from build123d import *

# Parameters (mm, degrees)
SKETCH1_W               = 72
SKETCH1_H               = 64
BOSS_EXTRUDE1_DEPTH     = 2.5
SKETCH2_R               = 3
BOSS_EXTRUDE2_DEPTH     = 11
CUT_EXTRUDE1_DEPTH      = 51.02249494
CUT_EXTRUDE1_DEPTH_BACK = 51.02249494
SKETCH3_R               = 1.5
FILLET1_R               = 5


with BuildPart() as part:
    # Sketch1 → Boss-Extrude1 (new body)
    with BuildSketch(Plane(origin=(0, 0, 0), x_dir=(1, 0, 0), z_dir=(0, 1, 0))):
        Rectangle(SKETCH1_W, SKETCH1_H)
    extrude(amount=BOSS_EXTRUDE1_DEPTH)

    # Sketch2 → Boss-Extrude2 (add)
    with BuildSketch(Plane(origin=(0, 2.5, 0), x_dir=(1, 0, 0), z_dir=(0, 1, 0))):
        with Locations(Location((-31, 27, 0), (0, 0, 270))):
            Circle(SKETCH2_R)
        with Locations(Location((26, 27, 0), (0, 0, 270))):
            Circle(SKETCH2_R)
        with Locations(Location((-31, -27, 0), (0, 0, 270))):
            Circle(SKETCH2_R)
        with Locations(Location((26, -27, 0), (0, 0, 270))):
            Circle(SKETCH2_R)
    extrude(amount=BOSS_EXTRUDE2_DEPTH)

    # Sketch3 → Cut-Extrude1 (cut, two sides: drawn at the far end of the back side and taken through both)
    with BuildSketch(Plane(origin=(0, 13.5, 0), x_dir=(1, 0, 0), z_dir=(0, 1, 0)).offset(-CUT_EXTRUDE1_DEPTH_BACK)):
        with Locations(Location((-31, 27, 0), (0, 0, 270))):
            Circle(SKETCH3_R)
        with Locations(Location((-31, -27, 0), (0, 0, 270))):
            Circle(SKETCH3_R)
        with Locations(Location((26, 27, 0), (0, 0, 270))):
            Circle(SKETCH3_R)
        with Locations(Location((26, -27, 0), (0, 0, 270))):
            Circle(SKETCH3_R)
    extrude(amount=CUT_EXTRUDE1_DEPTH + CUT_EXTRUDE1_DEPTH_BACK, mode=Mode.SUBTRACT)

    # Fillet1
    fillet1_edges = [part.edges().sort_by_distance(p)[0] for p in [
        (-36, 1.25, -32),
        (36, 1.25, -32),
        (36, 1.25, 32),
        (-36, 1.25, 32),
    ]]
    fillet(fillet1_edges, radius=FILLET1_R)


solid = part.part
Design review of the part built by this model. Coordinates are the model's own, in mm. A direction names the side the tool comes from. Coordinates: 2 decimals unless noted, no trailing zeros. Loops run counter-clockwise (first coordinate to the right, second up) from the corner with the lowest first, then second, coordinate; pieces in that order, holes last.
Item 1: Wall thickness on L1, parallel to X at y = 4, z = -27; L2, parallel to X at y = 1.25, z = -26; L3, parallel to Z at x = -30.5, y = 13.25: over which ranges is each line inside the solid? List them lowest first.
Completed:
L1: x = -34 to -32.5, -29.5 to -28, 23 to 24.5, 27.5 to 29
L2: x = -36 to -32.12, -29.88 to 24.88, 27.12 to 36
L3: z = -29.96 to -28.41, -25.59 to -24.04, 24.04 to 25.59, 28.41 to 29.96
Item 2: Add section A-A (y = 7). Write out the cut boundary in (x, z), and give its area (3 significant figures).
Completed:
outline: circle Ø6 at (-31, -27); circle Ø6 at (-31, 27); circle Ø6 at (26, -27); circle Ø6 at (26, 27); hole circle Ø3 at (-31, -27); hole circle Ø3 at (-31, 27); hole circle Ø3 at (26, -27); hole circle Ø3 at (26, 27)
area: 84.8 mm2
Item 3: Add section C-C (z = -19.5). Write out the cut boundary in (x, y), and give its area (3 significant figures).
Completed:
outline: (-36, 0) - (36, 0) - (36, 2.5) - (-36, 2.5) - close
area: 180 mm2
Item 4: Add section B-B (x = 26). Write out the cut boundary in (y, z), and give its area (3 significant figures).
Completed:
outline: (0, -32) - (2.5, -32) - (2.5, -30) - (13.5, -30) - (13.5, -28.5) - (0, -28.5) - close; (0, -25.5) - (13.5, -25.5) - (13.5, -24) - (2.5, -24) - (2.5, 24) - (13.5, 24) - (13.5, 25.5) - (0, 25.5) - close; (0, 28.5) - (13.5, 28.5) - (13.5, 30) - (2.5, 30) - (2.5, 32) - (0, 32) - close
area: 211 mm2
Item 5: For faces 1 (the cylindrical face through (26, 8, -30)), 2 (the cylindrical face through (27.01, 6.66, 25.89)), list the 3-axis set-ups (+Z, -Z, +X, -X, +Y, -Y) from which the entire face can be reached by the end or side of a thin tool; tool diameter is ignored.
Completed:
face 1: +Y
face 2: +Y, -Y
Item 6: Clearance check with flat-ended pins moving along their axes: pin 1 (6 mm diameter, centred on x = 20, z = 18.5, fed in from +Y); pin 2 (2 mm diameter, centred on y = 5, z = 11.5, fed in from +X); pin 3 (1 mm diameter, centred on y = 3.5, z = -24, fed in from -X). State where each tip first meets the part, or that it passes through.
Completed:
pin 1: stops at y = 2.5
pin 2: passes through
pin 3: stops at x = -32.66
Item 7: Draft analysis for pull direction X (two halves, no side actions). For faces 3 (the cylindrical face through (-30.93, 6.66, 25.5)), 4 (the flat face through (0, 1, 32)), 5 (the cylindrical face through (34, 1, -31)), state which applies: pulls with the +X half, pulls with the -X half, needs draft (parallel to the pull), parting line crosses it, or undercut.
Completed:
face 3: undercut
face 4: needs draft
face 5: pulls with the +X half
